Check sheet for the modelled part. Datum: model origin and axes. Units: mm. A direction names the side the tool comes from. Round coordinates to 2 decimals unless told otherwise and drop trailing zeros. Write each loop counter-clockwise with the first axis right and the second up, starting at its lowest first coordinate (ties: lowest second). Pieces come first, ordered by that corner, then holes. Notation, with made-up numbers: M -28,-23.75 L 15,-23.75 A29 cw 15,6.25 Z; hole C 69,16.25 d2. An arc over 180 degrees is marked long. Answer in a Markdown table with one row per item.
Autodesk Inventor part; units mm, degrees
ref_plane "YZ Plane" through (0, 0, 0) normal (1, 0, 0) x (0, 1, 0)
ref_plane "XZ Plane" through (0, 0, 0) normal (0, 1, 0) x (-1, 0, 0)
ref_plane "XY Plane" through (0, 0, 0) normal (0, 0, 1) x (1, 0, 0)
sketch "Sketch1" plane through (0, 0, 0) normal (0, 1, 0) x (-1, 0, 0)
  circle A0 centre (48.634, 12.202) radius 1.778
  circle A1 centre (29.509, 5.597) radius 1.778
  circle A2 centre (37, 18) radius 1.5
  circle A3 centre (21, 18) radius 1.5
  circle A4 centre (3, 13.5) radius 1.5
  circle A5 centre (21, 4) radius 1.5
  circle A6 centre (37, 4) radius 1.5
  circle A7 centre (55, 13.5) radius 1.5
  circle A8 centre (11.639, 12.326) radius 1.778
  circle A9 centre (20.363, 11.115) radius 1.778
  circle A10 centre (29.407, 12.701) radius 1.778
  circle A11 centre (38.211, 11.232) radius 1.778
  line L0 (10.2856, 4.4998) -> (-0.0002, 12.5003)
  line L1 (34.6899, 0.0005) -> (47.7142, 4.5002)
  line L2 (57.9997, 16.5) -> (40.0003, 16.5)
  line L3 (39.9997, 21) -> (17.9997, 21)
  line L4 (-0.0003, 16.5) -> (18.0003, 16.5)
  line L5 (10.2856, 4.4998) -> (23.0001, 0.0002)
  line L6 (47.7142, 4.5002) -> (57.9998, 12.5002)
  line L7 (57.9997, 16.5) -> (57.9998, 12.5002)
  line L8 (34.6899, 0.0005) -> (23.0001, 0.0002)
  line L9 (-0.0002, 12.5003) -> (-0.0003, 16.5)
  line L10 (18.0003, 16.5) -> (17.9997, 21)
  line L11 (39.9997, 21) -> (40.0003, 16.5)
  line L12 (51.9741, 15.2119) -> (45.332, 15.2119)
  line L13 (45.332, 15.2119) -> (45.332, 9.1159)
  line L14 (45.332, 9.1159) -> (51.9741, 9.1159)
  line L15 (51.9741, 9.1159) -> (51.9741, 15.2119)
  line L16 (41.259, 14.534) -> (35.2011, 14.534)
  line L17 (35.2011, 14.534) -> (35.2011, 7.93)
  line L18 (35.2011, 7.93) -> (41.259, 7.93)
  line L19 (41.259, 7.93) -> (41.259, 14.534)
  line L20 (32.7471, 15.7871) -> (26.105, 15.7871)
  line L21 (26.105, 15.7871) -> (26.105, 9.6911)
  line L22 (26.105, 9.6911) -> (32.7471, 9.6911)
  line L23 (32.7471, 9.6911) -> (32.7471, 15.7871)
  line L24 (32.8491, 8.6831) -> (26.207, 8.6831)
  line L25 (26.207, 8.6831) -> (26.207, 2.549)
  line L26 (26.207, 2.549) -> (32.8491, 2.549)
  line L27 (32.8491, 2.549) -> (32.8491, 8.6831)
  line L28 (23.4491, 14.417) -> (17.3531, 14.417)
  line L29 (17.3531, 14.417) -> (17.3531, 7.7749)
  line L30 (17.3531, 7.7749) -> (23.4491, 7.7749)
  line L31 (23.4491, 7.7749) -> (23.4491, 14.417)
  line L32 (14.9791, 15.4121) -> (8.337, 15.4121)
  line L33 (8.337, 15.4121) -> (8.337, 9.337)
  line L34 (8.337, 9.337) -> (14.9791, 9.337)
  line L35 (14.9791, 9.337) -> (14.9791, 15.4121)
  point P0 (0, 0)
extrude "Extrusion1" add sketch "Sketch1" along normal blind 1 contours A0 | A1 | A8 | A9 | A10 | A11 | L0 L9 L4 L10 L3 L11 L2 L7 L6 L1 L8 L5 | L15 L14 L13 L12 | L19 L18 L17 L16 | L23 L22 L21 L20 | L27 L26 L25 L24 | L31 L30 L29 L28 | L35 L34 L33 L32
extrude "Extrusion2" add sketch "Sketch1" against normal blind 3 contours L15 L14 L13 L12 | L19 L18 L17 L16 | L23 L22 L21 L20 | L27 L26 L25 L24 | L31 L30 L29 L28 | L35 L34 L33 L32
extrude "Extrusion3" add sketch "Sketch1" against normal blind 13 contours A0 | A1 | A8 | A9 | A10 | A11
ref_plane "Work Plane1" through (-28.9998, 0, 12.501) normal (1, 0, 0) x (0, 0, -1)
properties part number "Keyboard1"
1. Section check C-C, the plane z = 18. Record the cut outline in (x, y).
Found:
| item | result |
|---|---|
| outline | M -40,0 L -38.5,0 L -38.5,1 L -40,1 Z; M -35.5,0 L -22.5,0 L -22.5,1 L -35.5,1 Z; M -19.5,0 L -18,0 L -18,1 L -19.5,1 Z |
2. Access from +Z, -Z, +X, -X, +Y, -Y to the whole of each face (thin tool, end or side, straight path). Record for faces 5 (the face through (-56.43, 0.49, 13.05)), 6 (the face through (-32.747, -1, 13)), 7 (the face through (-17.353, -1, 11)), 8 (the face through (-51.974, -1, 12)), 9 (the face through (-19.98, -7.93, 9.38)).
Found:
| item | result |
|---|---|
| face 5 | +Y, -Y |
| face 6 | +Z, -Y |
| face 7 | +Z, -Z, -Y |
| face 8 | +Z, -Z, -X, -Y |
| face 9 | -Y |
3. Section check D-D, the plane x = -3. Record the cut outline in (y, z), and give its area (3 significant figures).
Found:
| item | result |
|---|---|
| outline | M 0,10.17 L 1,10.17 L 1,12 L 0,12 Z; M 0,15 L 1,15 L 1,16.5 L 0,16.5 Z |
| area | 3.33 mm2 |
4. Go/stop test with flat-tipped pins: pin 1 (1.5 mm diameter, centred on x = -10, y = -2, fed in from -Z); pin 2 (3.5 mm diameter, centred on y = -1.5, z = 11.5, fed in from +X); pin 3 (4 mm diameter, centred on x = -49.5, y = -1, fed in from +Z). Record where each tip stops, or that it passes through.
Found:
| item | result |
|---|---|
| pin 1 | stops at z = 9.34 |
| pin 2 | stops at x = -0.13 |
| pin 3 | stops at z = 16.5 |
5. Section check A-A, the plane y = -1. Record the cut outline in (x, z) (3 decimals).
Found:
| item | result |
|---|---|
| outline | M -51.974,9.116 L -45.332,9.116 L -45.332,15.212 L -51.974,15.212 Z; M -41.259,7.93 L -35.201,7.93 L -35.201,14.534 L -41.259,14.534 Z; M -32.849,2.549 L -26.207,2.549 L -26.207,8.683 L -32.849,8.683 Z; M -32.747,9.691 L -26.105,9.691 L -26.105,15.787 L -32.747,15.787 Z; M -23.449,7.775 L -17.353,7.775 L -17.353,14.417 L -23.449,14.417 Z; M -14.979,9.337 L -8.337,9.337 L -8.337,15.412 L -14.979,15.412 Z |
6. Draft check along X on faces 1 (the face through (-12, -13, 12)), 2 (the face through (-19, -3, 9.7)), 3 (the face through (-36.435, -7.93, 11.31)), 4 (the face through (-5.215, 0.493, 8.444)). Enter one of: +X half, -X half, draft (parallel to the pull), parting line (faces both ways), or undercut.
Found:
| item | result |
|---|---|
| face 1 | draft |
| face 2 | undercut |
| face 3 | undercut |
| face 4 | +X half |
7. Section check B-B, the plane x = -37.5. Record the cut outline in (y, z), and give its area (3 significant figures).
Found:
| item | result |
|---|---|
| outline | M -13,9.6 L -3,9.6 L -3,7.93 L 0,7.93 L 0,5.41 L 1,5.41 L 1,16.59 L 0,16.59 L 0,14.53 L -3,14.53 L -3,12.86 L -13,12.86 Z; M 0,0.97 L 1,0.97 L 1,2.59 L 0,2.59 Z; M 0,19.41 L 1,19.41 L 1,21 L 0,21 Z |
| area | 66.8 mm2 |
8. Scan lines: L1, parallel to Z at x = -37, y = 0.85; L2, parallel to Z at x = -21, y = 0.35; L3, parallel to Y at x = -7.5, z = 12. Record each from-to range of solid material in increasing order.
Found:
| item | result |
|---|---|
| L1 | z = 0.8 to 2.5, 5.5 to 16.5, 19.5 to 21 |
| L2 | z = 0.71 to 2.5, 5.5 to 16.5, 19.5 to 21 |
| L3 | y = 0 to 1 |
